```python
from build123d import *

# Parameters (mm, degrees)
BOSS_EXTRUDE1_DEPTH                                 = 10
CSK_FOR_M2_COUNTERSUNK_FLAT_HEAD_SCREW1_D           = 2.4
CSK_FOR_M2_COUNTERSUNK_FLAT_HEAD_SCREW1_DEPTH       = 30
CSK_FOR_M2_COUNTERSUNK_FLAT_HEAD_SCREW1_CSINK_D     = 4.4
CSK_FOR_M2_COUNTERSUNK_FLAT_HEAD_SCREW1_CSINK_ANGLE = 90
CSK_FOR_M2_COUNTERSUNK_FLAT_HEAD_SCREW1_TIP         = 0.721032743
SKETCH4_R                                           = 1
CUT_EXTRUDE1_DEPTH                                  = 91.691785736
SKETCH5_R                                           = 2
CUT_EXTRUDE2_DEPTH                                  = 88.27685833
FILLET1_R                                           = 1


with BuildPart() as part:
    # Sketch1 → Boss-Extrude1 (new body)
    with BuildSketch(Plane(origin=(0, 0, 0), x_dir=(0, 0, -1), z_dir=(1, 0, 0))):
        Polygon((0, 0), (0, 75), (-6.5, 75), (-6.5, 6.5), (-50, 6.5), (-50, 0), align=None)
    extrude(amount=BOSS_EXTRUDE1_DEPTH)

    # CSK for M2 Countersunk Flat Head Screw1
    with Locations(Plane(origin=(0, 6.5, 0), x_dir=(1, 0, 0), z_dir=(0, 1, 0))):
        with Locations((5, -28.25)):
            CounterSinkHole(CSK_FOR_M2_COUNTERSUNK_FLAT_HEAD_SCREW1_D / 2, CSK_FOR_M2_COUNTERSUNK_FLAT_HEAD_SCREW1_CSINK_D / 2, depth=CSK_FOR_M2_COUNTERSUNK_FLAT_HEAD_SCREW1_DEPTH, counter_sink_angle=CSK_FOR_M2_COUNTERSUNK_FLAT_HEAD_SCREW1_CSINK_ANGLE)
            with Locations((0, 0, -(CSK_FOR_M2_COUNTERSUNK_FLAT_HEAD_SCREW1_DEPTH + CSK_FOR_M2_COUNTERSUNK_FLAT_HEAD_SCREW1_TIP / 2))):  # 118° drill point
                Cone(0, CSK_FOR_M2_COUNTERSUNK_FLAT_HEAD_SCREW1_D / 2, CSK_FOR_M2_COUNTERSUNK_FLAT_HEAD_SCREW1_TIP, mode=Mode.SUBTRACT)

    # Sketch4 → Cut-Extrude1 (cut, through all)
    with BuildSketch(Plane.ZY):
        with Locations((3.370981866, 33.7)):
            Circle(SKETCH4_R)
        with Locations((3.370981866, 43.6)):
            Circle(SKETCH4_R)
    extrude(amount=-CUT_EXTRUDE1_DEPTH, mode=Mode.SUBTRACT)

    # Sketch5 → Cut-Extrude2 (cut, through all)
    with BuildSketch(Plane.XY.offset(6.5)):
        with Locations((5, 43.61)):
            Circle(SKETCH5_R)
        with Locations((5, 33.71)):
            Circle(SKETCH5_R)
    extrude(amount=-CUT_EXTRUDE2_DEPTH, mode=Mode.SUBTRACT)

    # Fillet1
    fillet1_edges = [part.edges().sort_by_distance(p)[0] for p in [
        (5, 0, 50),
        (5, 6.5, 50),
        (5, 6.5, 6.5),
        (5, 75, 6.5),
        (5, 75, 0),
        (5, 0, 0),
        (10, 75, 3.25),
        (10, 40.75, 6.5),
        (10, 6.5, 28.25),
        (10, 3.25, 50),
        (10, 0, 25),
        (0, 3.25, 50),
        (0, 6.5, 28.25),
        (0, 40.75, 6.5),
        (0, 75, 3.25),
        (0, 37.5, 0),
        (0, 0, 25),
        (10, 37.5, 0),
    ]]
    fillet(fillet1_edges, radius=FILLET1_R)


solid = part.part
```
Model file for the job. Use its own axes, mm. A direction names the side the tool comes from. Coordinates: 2 decimals unless noted, no trailing zeros. Write each loop counter-clockwise with the first axis right and the second up, starting at its lowest first coordinate (ties: lowest second). Pieces come first, ordered by that corner, then holes. Notation, with made-up numbers: (27.5, 79) - (38.5, 79) arc R12 cw to (38.5, 85) - close; hole circle Ø4 at (0.25, 9). An arc over 180 degrees is marked (long way). Use a Markdown table: item, result. Add a question column.
Item 1: Band-saw the part on B-B, the plane z = 28.25. Write the cut outline in (x, y).
Item 2: Drop flat-ended pins along their axis: pin 1 (3 mm diameter, centred on x = 5, z = 28.25, fed in from +Y); pin 2 (1.2 mm diameter, centred on y = 43.6, z = 3.37, fed in from -X); pin 3 (8 mm diameter, centred on y = 10, z = 33.5, fed in from +X); pin 4 (2.5 mm diameter, centred on x = 3.5, y = 38, fed in from +Z). Give the stop position or say it passes through.
Item 3: Band-saw the part on A-A, the plane x = 5. Write the cut outline in (y, z), and give its area (3 significant figures).
Item 4: Band-saw the part on C-C, the plane y = 15. Write the cut outline in (x, z), and give its area (3 significant figures).
Item 5: Two-plate mould, pull along Z, no slides. Class faces 3 (the face through (5, 41, 6.5)), 4 (the face through (8.34, 33.317, 4.295)), 5 (the face through (5, 75, 3)): pulls with the +Z half, pulls with the -Z half, needs draft (parallel to the pull), parting line crosses it, or undercut.
Item 6: Drill centre lines: line 1 along Y through (x, z) = (5, 4.75); line 2 along X through (y, z) = (3.7, 28.25); line 3 along Z through (x, y) = (9.05, 33.7). Where is each one in solid material? Low to high.
Item 7: 3-axis set-ups, long thin cutter, end or side, ignore diameter. For faces 1 (the face through (2, 6.5, 28)), 2 (the face through (5, 0, 25)): which of +Z, -Z, +X, -X, +Y, -Y reach the whole face in a straight line?
A:
| question | item | result |
|---|---|---|
| 1 | outline | (0, 1) arc R1 ccw to (1, 0) - (3.8, 0) - (3.8, 5.5) - (2.8, 6.5) - (1, 6.5) arc R1 ccw to (0, 5.5) - close; (6.2, 0) - (9, 0) arc R1 ccw to (10, 1) - (10, 5.5) arc R1 ccw to (9, 6.5) - (7.2, 6.5) - (6.2, 5.5) - close |
| 2 | pin 1 | stops at y = 5.8 |
| 2 | pin 2 | passes through |
| 2 | pin 3 | stops at x = 9.87 |
| 2 | pin 4 | stops at z = 6.5 |
| 3 | outline | (0, 1) arc R1 ccw to (1, 0) - (31.71, 0) - (31.71, 6.5) - (7.5, 6.5) arc R1 cw to (6.5, 7.5) - (6.5, 26.05) - (5.5, 27.05) - (0, 27.05) - close; (0, 29.45) - (5.5, 29.45) - (6.5, 30.45) - (6.5, 49) arc R1 ccw to (5.5, 50) - (1, 50) arc R1 ccw to (0, 49) - close; (35.71, 0) - (41.61, 0) - (41.61, 6.5) - (35.71, 6.5) - close; (45.61, 0) - (74, 0) arc R1 ccw to (75, 1) - (75, 5.5) arc R1 ccw to (74, 6.5) - (45.61, 6.5) - close |
| 3 | area | 701 mm² |
| 4 | outline | (0, 1) arc R1 ccw to (1, 0) - (9, 0) arc R1 ccw to (10, 1) - (10, 5.5) arc R1 ccw to (9, 6.5) - (1, 6.5) arc R1 ccw to (0, 5.5) - close |
| 4 | area | 64.1 mm² |
| 5 | face 3 | pulls with the +Z half |
| 5 | face 4 | undercut |
| 5 | face 5 | needs draft |
| 6 | line 1 | y = 0 to 31.71, 35.71 to 41.61, 45.61 to 75 |
| 6 | line 2 | x = 0 to 3.8, 6.2 to 10 |
| 6 | line 3 | z = 0 to 2.37, 4.37 to 6.5 |
| 7 | face 1 | +Z, +X, -X, +Y |
| 7 | face 2 | +Z, -Z, +X, -X, -Y |
